The listing builds one solid part. Answer for the finished solid, in the listing's coordinates (mm). A direction names the side the tool comes from. Round coordinates to 2 decimals unless told otherwise and drop trailing zeros. Write each loop counter-clockwise with the first axis right and the second up, starting at its lowest first coordinate (ties: lowest second). Pieces come first, ordered by that corner, then holes. Notation, with made-up numbers: (-38.5, 87) - (-30.5, 87) arc R20 ccw to (-30.5, 126) - close; hole circle Ø5 at (-23.5, -22). An arc over 180 degrees is marked (long way). Answer in a Markdown table with one row per item.
from build123d import *
from build123d.topology import SkipClean

# Parameters (mm, degrees)
BASE_EXTRUDE_DEPTH   = 1.9685
SKETCH2_R            = 2.3876
CUT_EXTRUDE1_DEPTH   = 17.830524964
SKETCH3_R            = 3.048
CUT_EXTRUDE2_DEPTH   = 1.143
CUT_EXTRUDE3_START   = -1.143
SKETCH4_R            = 3.048
CUT_EXTRUDE3_DEPTH   = 1.143
LPATTERN1_COUNT      = 2
LPATTERN1_PITCH      = 7.9375
CUT_EXTRUDE4_DEPTH   = 17.830524964
FILLET1_R            = 0.396875
CUT_EXTRUDE5_DEPTH   = 17.830524964
FILLET2_R            = 0.1984375
FILLET1_OF_MIRROR1_R = 0.396875
FILLET2_OF_MIRROR1_R = 0.1984375
CUT_EXTRUDE6_DEPTH   = 1.143
FILLET3_R            = 0.1984375
FILLET3_OF_MIRROR2_R = 0.1984375
SKETCH8_R            = 3.96875
SKETCH8_R_2          = 2.3876
BOSS_EXTRUDE1_DEPTH  = 3.937
CUT_EXTRUDE7_START   = -3.937
SKETCH9_R            = 2.3876
CUT_EXTRUDE7_DEPTH   = 3.937
CIRPATTERN1_COUNT    = 4


with BuildPart() as part:
    # Sketch1 → Base-Extrude (new, symmetric)
    with BuildSketch(Plane(origin=(0, 0, 0), x_dir=(1, 0, 0), z_dir=(0, 1, 0))):
        with BuildLine():
            Line((-11.90625, 3.96875), (11.90625, 3.96875))
            ThreePointArc((11.90625, 3.96875), (15.875, 0), (11.90625, -3.96875))
            Line((11.90625, -3.96875), (-11.90625, -3.96875))
            ThreePointArc((-11.90625, -3.96875), (-15.875, 0), (-11.90625, 3.96875))
        make_face()
    extrude(amount=BASE_EXTRUDE_DEPTH, both=True)

    # Sketch2 → Cut-Extrude1 (cut, through all)
    with BuildSketch(Plane(origin=(0, 1.9685, 0), x_dir=(-1, 0, 0), z_dir=(0, 1, 0))):
        with Locations(Location((3.96875, 0, 0), (0, 0, 90))):
            Circle(SKETCH2_R)
    cut_extrude1 = extrude(amount=-CUT_EXTRUDE1_DEPTH, mode=Mode.SUBTRACT)

    # Sketch3 → Cut-Extrude2 (cut)
    with BuildSketch(Plane(origin=(0, 1.9685, 0), x_dir=(-1, 0, 0), z_dir=(0, 1, 0))):
        with Locations(Location((3.96875, 0, 0), (0, 0, 90))):
            Circle(SKETCH3_R)
    cut_extrude2 = extrude(amount=-CUT_EXTRUDE2_DEPTH, mode=Mode.SUBTRACT)

    # Sketch4 → Cut-Extrude3 (cut)
    with BuildSketch(Plane.XZ.offset(1.9685).offset(CUT_EXTRUDE3_START)):
        with Locations(Location((-3.96875, 0, 0), (0, 0, 90))):
            Circle(SKETCH4_R)
    cut_extrude3 = extrude(amount=CUT_EXTRUDE3_DEPTH, mode=Mode.SUBTRACT)

    # LPattern1: Cut-Extrude1, Cut-Extrude2, Cut-Extrude3 ×2
    with Locations(*[(i * LPATTERN1_PITCH, 0, 0) for i in range(1, LPATTERN1_COUNT)]):
        add(cut_extrude1, mode=Mode.SUBTRACT)
        add(cut_extrude2, mode=Mode.SUBTRACT)
        add(cut_extrude3, mode=Mode.SUBTRACT)

    # Sketch5 → Cut-Extrude4 (cut, through all)
    with BuildSketch(Plane(origin=(0, 1.9685, 0), x_dir=(-1, 0, 0), z_dir=(0, 1, 0))):
        with BuildLine():
            Line((10.9855, -2.202919244), (10.9855, -0.92075))
            Line((10.9855, -0.92075), (9.703330756, -0.92075))
            ThreePointArc((9.703330756, -0.92075), (9.51865, 0), (9.703330756, 0.92075))
            Line((9.703330756, 0.92075), (10.9855, 0.92075))
            Line((10.9855, 0.92075), (10.9855, 2.202919244))
            ThreePointArc((10.9855, 2.202919244), (11.90625, 2.3876), (12.827, 2.202919244))
            Line((12.827, 2.202919244), (12.827, 0.92075))
            Line((12.827, 0.92075), (14.109169244, 0.92075))
            ThreePointArc((14.109169244, 0.92075), (14.29385, 0), (14.109169244, -0.92075))
            Line((14.109169244, -0.92075), (12.827, -0.92075))
            Line((12.827, -0.92075), (12.827, -2.202919244))
            ThreePointArc((12.827, -2.202919244), (11.90625, -2.3876), (10.9855, -2.202919244))
        make_face()
    cut_extrude4 = extrude(amount=-CUT_EXTRUDE4_DEPTH, mode=Mode.SUBTRACT)

    # Fillet1
    fillet1_edges = [part.edges().sort_by_distance(p)[0] for p in [
        (-10.9855, 0, 0.92075),
        (-12.827, 0, 0.92075),
        (-12.827, 0, -0.92075),
        (-10.9855, 0, -0.92075),
    ]]
    fillet(fillet1_edges, radius=FILLET1_R)

    # Sketch6 → Cut-Extrude5 (cut, through all)
    with BuildSketch(Plane(origin=(0, 1.9685, 0), x_dir=(-1, 0, 0), z_dir=(0, 1, 0))):
        with BuildLine():
            Line((9.271007651, -2.3876), (6.603992349, -2.3876))
            ThreePointArc((6.603992349, -2.3876), (7.52475, 0), (6.603992349, 2.3876))
            Line((6.603992349, 2.3876), (9.271007651, 2.3876))
            ThreePointArc((9.271007651, 2.3876), (8.783903639, 1.701789999), (8.471522145, 0.92075))
            Line((8.471522145, 0.92075), (9.703330756, 0.92075))
            ThreePointArc((9.703330756, 0.92075), (9.51865, 0), (9.703330756, -0.92075))
            Line((9.703330756, -0.92075), (8.471522145, -0.92075))
            ThreePointArc((8.471522145, -0.92075), (8.783903639, -1.701789999), (9.271007651, -2.3876))
        make_face()
    cut_extrude5 = extrude(amount=-CUT_EXTRUDE5_DEPTH, mode=Mode.SUBTRACT)

    # Fillet2
    fillet2_edges = [part.edges().sort_by_distance(p)[0] for p in [
        (-8.471522145, 0, -0.92075),
        (-9.271007651, 0, -2.3876),
        (-6.603992349, 0, -2.3876),
        (-6.603992349, 0, 2.3876),
        (-9.271007651, 0, 2.3876),
        (-8.471522145, 0, 0.92075),
    ]]
    fillet(fillet2_edges, radius=FILLET2_R)

    # Mirror1: Cut-Extrude4, Cut-Extrude5 across plane
    add(cut_extrude4.mirror(Plane(origin=(0, 0, 0), x_dir=(0, 0, 1), z_dir=(1, 0, 0))), mode=Mode.SUBTRACT)
    add(cut_extrude5.mirror(Plane(origin=(0, 0, 0), x_dir=(0, 0, 1), z_dir=(1, 0, 0))), mode=Mode.SUBTRACT)

    # Fillet1 of Mirror1
    fillet1_of_mirror1_edges = [part.edges().sort_by_distance(p)[0] for p in [
        (10.9855, 0, 0.92075),
        (12.827, 0, 0.92075),
        (12.827, 0, -0.92075),
        (10.9855, 0, -0.92075),
    ]]
    fillet(fillet1_of_mirror1_edges, radius=FILLET1_OF_MIRROR1_R)

    # Fillet2 of Mirror1
    fillet2_of_mirror1_edges = [part.edges().sort_by_distance(p)[0] for p in [
        (8.471522145, 0, -0.92075),
        (9.271007651, 0, -2.3876),
        (6.603992349, 0, -2.3876),
        (6.603992349, 0, 2.3876),
        (9.271007651, 0, 2.3876),
        (8.471522145, 0, 0.92075),
    ]]
    fillet(fillet2_of_mirror1_edges, radius=FILLET2_OF_MIRROR1_R)

    # Sketch7 → Cut-Extrude6 (cut)
    with BuildSketch(Plane(origin=(7.626637742, 1.9685, -1.750590375), x_dir=(-1, 0, 0), z_dir=(0, 1, 0))):
        with BuildLine():
            Line((8.960145393, -0.637009625), (6.293130092, -0.637009625))
            ThreePointArc((6.293130092, -0.637009625), (7.213887742, 1.750590375), (6.293130092, 4.138190375))
            Line((6.293130092, 4.138190375), (8.960145393, 4.138190375))
            ThreePointArc((8.960145393, 4.138190375), (8.277552771, 3.030085237), (8.039387742, 1.750590375))
            ThreePointArc((8.039387742, 1.750590375), (8.277552771, 0.471095513), (8.960145393, -0.637009625))
        make_face()
    cut_extrude6 = extrude(amount=-CUT_EXTRUDE6_DEPTH, mode=Mode.SUBTRACT)

    # Fillet3
    fillet3_edges = [part.edges().sort_by_distance(p)[0] for p in [
        (-1.333507651, 1.397, -2.3876),
        (1.333507651, 1.397, -2.3876),
        (1.333507651, 1.397, 2.3876),
        (-1.333507651, 1.397, 2.3876),
    ]]
    fillet(fillet3_edges, radius=FILLET3_R)

    # Mirror2: Cut-Extrude6 across plane
    add(cut_extrude6.mirror(Plane.ZX), mode=Mode.SUBTRACT)

    # Fillet3 of Mirror2
    fillet3_of_mirror2_edges = [part.edges().sort_by_distance(p)[0] for p in [
        (-1.333507651, -1.397, -2.3876),
        (1.333507651, -1.397, -2.3876),
        (1.333507651, -1.397, 2.3876),
        (-1.333507651, -1.397, 2.3876),
    ]]
    fillet(fillet3_of_mirror2_edges, radius=FILLET3_OF_MIRROR2_R)

    # Sketch8 → Boss-Extrude1 (add)
    with SkipClean():  # the faces are left unmerged after this step: merging them gives an invalid solid
        with BuildSketch(Plane.XZ.offset(1.9685)):
            with Locations(Location((11.90625, 0, 0), (0, 0, 270))):
                Circle(SKETCH8_R)
            with Locations(Location((11.90625, 0, 0), (0, 0, 67.31662771))):
                Circle(SKETCH8_R_2, mode=Mode.SUBTRACT)
        extrude(amount=BOSS_EXTRUDE1_DEPTH)

    # Sketch9 → Cut-Extrude7 (cut)
    with SkipClean():  # the faces are left unmerged after this step: merging them gives an invalid solid
        with BuildSketch(Plane.XZ.offset(5.9055).offset(CUT_EXTRUDE7_START)):
            with Locations((15.875, -3.96875)):
                Circle(SKETCH9_R)
        cut_extrude7 = extrude(amount=CUT_EXTRUDE7_DEPTH, mode=Mode.SUBTRACT)

    # CirPattern1: Cut-Extrude7 ×4 about axis
    with SkipClean():  # the faces are left unmerged after this step: merging them gives an invalid solid
        cirpattern1_axis = Axis((11.90625, 0, 0), (0, 1, 0))
        for i in range(1, CIRPATTERN1_COUNT):
            add(cut_extrude7.rotate(cirpattern1_axis, i * 360 / CIRPATTERN1_COUNT), mode=Mode.SUBTRACT)


solid = part.part
(1) Find the intervals of material crossed by line 1 (X direction, y = -1.4, z = 0) (3 decimals); line 2 (X direction, y = 0, z = 0) (3 decimals); line 3 (Y direction, x = 2, z = -3.5), in increasing order.
Checked values:
| item | result |
|---|---|
| line 1 | x = -15.875 to -14.294, -7.525 to -7.017, -0.921 to -0.413, 0.413 to 0.921, 7.017 to 7.525, 14.294 to 15.875 |
| line 2 | x = -15.875 to -14.294, -7.525 to -6.356, -1.581 to 1.581, 6.356 to 7.525, 14.294 to 15.875 |
| line 3 | y = -1.97 to 1.97 |
(2) For a pull along Z with two mould halves and no side action, classify faces 4 (the cylindrical face through (-8.757, 0.028, 1.652)), 5 (the flat face through (10, -5.906, 2)), 6 (the cylindrical face through (14.2, -3.91, -2.27)) as pulls with the +Z half, pulls with the -Z half, needs draft (parallel to the pull), parting line crosses it, or undercut.
Checked values:
| item | result |
|---|---|
| face 4 | undercut |
| face 5 | needs draft |
| face 6 | pulls with the -Z half |
(3) Section A-A (y = -4.25) is taken. Give the vertices of the cut face in (x, z) (1 decimal).
Checked values:
| item | result |
|---|---|
| outline | (8.3, -1.6) arc R2.4 cw to (10.3, -3.6) arc R4 ccw to (13.5, -3.6) arc R2.4 cw to (15.5, -1.6) arc R4 ccw to (15.5, 1.6) arc R2.4 cw to (13.5, 3.6) arc R4 ccw to (10.3, 3.6) arc R2.4 cw to (8.3, 1.6) arc R4 ccw to start; hole circle Ø4.8 at (11.9, 0) |
(4) Flat-ended cylindrical pins translate along their axes: pin 1 (1.1 mm diameter, centred on x = 7.5, z = 3, fed in from -Y); pin 2 (1.8 mm diameter, centred on x = -3, z = -1, fed in from -Y); pin 3 (2 mm diameter, centred on y = 0.5, z = -1.5, fed in from -X); pin 4 (1 mm diameter, centred on x = 14, y = -0.5, fed in from +Z). Find the tip coordinate at first contact, or state that the pin passes through.
Checked values:
| item | result |
|---|---|
| pin 1 | stops at y = -1.97 |
| pin 2 | passes through |
| pin 3 | stops at x = -15.84 |
| pin 4 | stops at z = 3.63 |
(5) For faces 1 (the cylindrical face through (-8.75, 0.03, -1.64)), 2 (the flat face through (13.3, -1.968, -1.4)), 3 (the cylindrical face through (8.75, 0.03, -1.64)), determine the directions among +Z, -Z, +X, -X, +Y, -Y from which every point of the face is accessible in a straight line to the end or side of a thin tool.
Checked values:
| item | result |
|---|---|
| face 1 | +Y, -Y |
| face 2 | -Y |
| face 3 | +Y |
(6) Section B-B (y = -1.25) is taken. State how many separate pieces and enclosed holes the cut face has, and give its area (3 significant figures).
Checked values:
| item | result |
|---|---|
| separate pieces | 1 |
| enclosed holes | 5 |
| area | 128 mm2 |
